Autodesk Inventor part; units mm, degrees
ref_plane "Work Plane1" through (0, 4.3647, 0.1782) normal (0, 0.9991679, 0.0407857) x (-1, 0, 0)
ref_plane "Work Plane2" through (0, -5.1058, 24.4292) normal (0, 0, 1) x (1, 0, 0)
ref_plane "Work Plane3" through (0, -4.3311, -22.2941) normal (0, 0, 1) x (1, 0, 0)
sketch "Sketch3" plane through (0, 0, 0) normal (1, 0, 0) x (0, 1, 0)
  arc A0 (-1.1214, 20.6041) -> (-9.0936, 20.4414) centre (-5.1058, 20.4414) ccw
  circle A1 centre (-5.1058, 20.4414) radius 1.524
  arc A2 (-9.0936, -17.5316) -> (0.4274, -17.3373) centre (-4.3311, -17.5316) ccw
  circle A3 centre (-4.3311, -17.5316) radius 1.524
  arc A4 (-0.102, -4.3672) -> (-0.4576, 4.3443) centre (0, 0) ccw
  circle A5 centre (0, 0) radius 1.4605
  line L0 (-9.0936, 20.4414) -> (-9.0936, -17.5316)
  line L1 (-1.1214, 20.6041) -> (-0.4576, 4.3443)
  line L2 (-0.102, -4.3672) -> (0.4274, -17.3373)
  line L3 (0, 0) -> (0, 35.9976) construction
  line L4 (0, 0) -> (20.0348, 0) construction
  line L5 (9.2339, 18.9174) -> (-10.5183, 18.9174) construction
  line L6 (11.5384, -16.0076) -> (-16.1147, -16.0076) construction
  line L7 (4.3684, 5.3055) -> (4.3684, -5.6899) construction
  line L8 (-1.4605, 3.5835) -> (-1.4605, -5.6899) construction
  dimension "d5" = 2.921
  dimension "d38" = 3.048
  dimension "d39" = 3.9878
  dimension "d40" = 4.7625
  dimension "d41" = 34.925
  dimension "d42" = 13.462
  dimension "d43" = 8.636
  dimension "d44" = 8.9916
  dimension "d45" = 7.6331
extrude "Extrusion1" add sketch "Sketch3" along normal mid plane 45.72
ref_plane "Work Plane1" through (0, 4.3647, 0.1782) normal (0, 0.9991679, 0.0407857) x (-1, 0, 0)
sketch "Sketch5" plane through (0, 4.3647, 0.1782) normal (0, 0.9991679, 0.0407857) x (-1, 0, 0)
  line L0 (-22.86, -7.8915) -> (-22.86, 24.6205)
  line L1 (-22.86, 24.6205) -> (-18.288, 24.6205)
  line L2 (-18.288, 24.6205) -> (-18.288, 4.3594)
  line L3 (-18.288, 4.3594) -> (-22.86, -7.8915)
  line L4 (-22.86, 20.6327) -> (-22.86, 4.3594)
  line L5 (22.86, 0) -> (-22.86, 0)
  line L6 (22.86, 24.6205) -> (-22.86, 24.6205)
  line L7 (22.86, 4.3594) -> (-22.86, 4.3594)
  line L8 (-22.86, 4.3594) -> (-22.86, -4.3594)
  line L9 (22.86, -4.3594) -> (-22.86, -4.3594)
  line L10 (22.86, -4.3594) -> (22.86, 4.3594)
  line L11 (22.86, 4.3594) -> (-22.86, 4.3594)
  line L12 (22.86, 24.6205) -> (22.86, -8.3995)
  line L13 (22.86, -8.3995) -> (9.398, 4.3594)
  line L14 (9.398, 4.3594) -> (9.398, 24.6205)
  line L15 (22.86, -22.1028) -> (-22.86, -22.1028)
  line L16 (14.986, -9.6568) -> (-14.986, -9.6568)
  line L17 (-14.986, -9.6568) -> (-14.986, -22.1028)
  line L18 (-14.986, -22.1028) -> (14.986, -22.1028)
  line L19 (14.986, -22.1028) -> (14.986, -9.6568)
  line L20 (3.556, 14.4605) -> (-12.446, 14.4605)
  line L21 (-12.446, 14.4605) -> (-12.446, 24.6205)
  line L22 (-12.446, 24.6205) -> (3.556, 24.6205)
  line L23 (3.556, 24.6205) -> (3.556, 14.4605)
  line L24 (-22.86, -4.3594) -> (-22.86, -17.3403)
  line L25 (22.86, -17.3403) -> (22.86, -4.3594)
  line L26 (-8.128, 4.3594) -> (-0.254, 4.3594)
  line L27 (-0.254, 4.3594) -> (-0.254, -4.3594)
  line L28 (-0.254, -4.3594) -> (-8.128, -4.3594)
  line L29 (-8.128, -4.3594) -> (-8.128, 4.3594)
  point P0 (0, 0)
  dimension "d21" = 32.512
  dimension "d22" = 4.572
  dimension "d26" = 33.02
  dimension "d27" = 5.842
  dimension "d28" = 5.842
  dimension "d29" = 10.16
  dimension "d31" = 12.446
  dimension "d32" = 7.874
  dimension "d33" = 7.874
  dimension "d34" = 10.16
  dimension "d36" = 29.972
  dimension "d37" = 16.002
extrude "Extrusion2" cut sketch "Sketch5" against normal up to surface contours L0 L9 L3 | L0 L5 L3 L9 | L0 L7 L3 L5 | L29 L5 L27 L9 | L0 L1 L2 L7 | L29 L7 L27 L5 | L13 L5 L10 L9 | L9 L12 L13 | L6 L23 L20 L21 | L13 L7 L10 L5 | L14 L6 L12 L7 | L15 L17 L16 L19 surface through (0, -9.0936, -17.5316) normal (0, -1, 0)
ref_plane "Work Plane2" through (0, -5.1058, 24.4292) normal (0, 0, 1) x (1, 0, 0)
ref_plane "Work Plane3" through (0, -4.3311, -22.2941) normal (0, 0, 1) x (1, 0, 0)
properties part number "Transmission Plate - Top"
Here's how the part is built. I have some questions about the finished solid (model axes, mm). A direction names the side the tool comes from. Round coordinates to 2 decimals unless told otherwise and drop trailing zeros. Loops run counter-clockwise (first coordinate to the right, second up) from the corner with the lowest first, then second, coordinate; pieces in that order, holes last.
1. Suppose I cut it at C-C, the plane y = -7.25. Please give me the cut outline in (x, z).
Answers:
outline: (-22.86, -21.29) - (-14.99, -21.29) - (-14.99, -9.96) - (14.99, -9.96) - (14.99, -21.29) - (22.86, -21.29) - (22.86, -8.19) - (18.29, 4.07) - (18.29, 23.8) - (12.45, 23.8) - (12.45, 14.18) - (-3.56, 14.18) - (-3.56, 23.8) - (-9.4, 23.8) - (-9.4, 4.07) - (-22.86, -8.7) - close; hole (0.25, -4.66) - (8.13, -4.66) - (8.13, 4.07) - (0.25, 4.07) - close
2. Thinking about a two-plate mould opening in Z: for faces 3 (the face through (-3.556, -5, 18)), 4 (the face through (15.326, -5.274, 24.426)), 5 (the face through (15.33, -5.44, 21.93)), which applies, released by +Z, released by -Z, zero draft, split by the parting line, or undercut?
Answers:
face 3: zero draft
face 4: released by +Z
face 5: undercut
3. Suppose I cut it at D-D, the plane x = 11. Please give me the cut outline in (y, z).
Answers:
outline: (-9.09, -10.04) - (0.11, -9.66) - (-0.1, -4.37) arc R4.37 ccw (long way) to (-0.46, 4.34) - (-0.87, 14.44) - (-9.09, 14.1) - close; hole circle Ø2.92 at (0, 0)
4. For faces 1 (the face through (-6.518, -5.274, 24.426)), 2 (the face through (-0.3, 0.1, -9.3)), which set-ups out of +Z, -Z, +X, -X, +Y, -Y let a thin tool reach every point of the face, with its end or its side?
Answers:
face 1: +Z, +X, -X
face 2: +X, -X, +Y
5. Will these pins go through, and if not, where does the flat tip stop? pin 1 (6.5 mm diameter, centred on y = -3.5, z = 20.5, fed in from -X); pin 2 (2 mm diameter, centred on x = -13, y = -3.5, fed in from -Z); pin 3 (5 mm diameter, centred on x = -2.5, z = 4, fed in from +Y).
Answers:
pin 1: stops at x = -9.4
pin 2: stops at z = -9.85
pin 3: stops at y = 4.1
6. If I drill on probe 1 along X at (y, z) = (-3.25, -12); probe 2 along Y at (x, z) = (11, 0); probe 3 along X at (y, z) = (-7.25, 6.5), over which ranges is the centre line in solid material (lowest first)?
Answers:
probe 1: x = -22.86 to -14.99, 14.99 to 22.86
probe 2: y = -9.09 to -1.46, 1.46 to 4.37
probe 3: x = -9.4 to 18.29
7. Suppose I cut it at B-B, the plane z = -2.5. Please give me the cut outline in (x, y), and give its area (3 significant figures).
Answers:
outline: (-16.79, 3.58) - (-16.24, -9.09) - (0.25, -9.09) - (0.25, 3.58) - close; (8.13, -9.09) - (20.71, -9.09) - (20.9, 3.58) - (8.13, 3.58) - close
area: 373 mm2
